CAD build for the part. Positions are in the model's coordinates, mm. Face numbers are marked on the shaded views. A direction names the side the tool comes from. Coordinates: 2 decimals unless noted, no trailing zeros. Loops run counter-clockwise (first coordinate to the right, second up) from the corner with the lowest first, then second, coordinate; pieces in that order, holes last. Notation, with made-up numbers: (-13, -13) - (40, -13) arc R21 ccw to (40, 25) - close; hole circle Ø11 at (-35.75, -5.5). An arc over 180 degrees is marked (long way). Put each result on its own line as item: value.
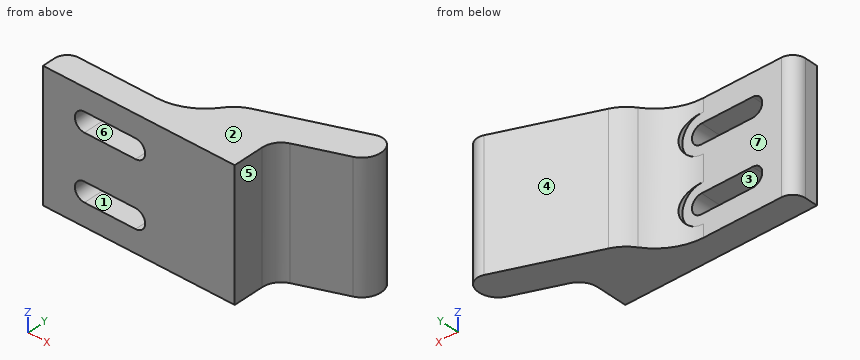
```python
from build123d import *

# Parameters (mm, degrees)
F2_DEPTH = 10
F4_DEPTH = 25
F6_DEPTH = 25


with BuildPart() as f2:
    # F1 (on Top) → F2 (new body, symmetric)
    with BuildSketch(Plane.XY):
        with BuildLine():
            Line((-41.03757, 2), (-41.03757, 0))
            Line((-41.03757, 0), (-11.03757, 0))
            Line((-11.03757, 0), (-11.03757, 4.786366))
            ThreePointArc((-11.03757, 4.786366), (-10.519333, 6.471849), (-9.143667, 7.575012))
            Line((-9.143667, 7.575012), (-1.893904, 10.450577))
            ThreePointArc((-1.893904, 10.450577), (-0.246001, 12.049481), (-0.211353, 14.34532))
            ThreePointArc((-0.211353, 14.34532), (-1.277289, 15.443922), (-2.807848, 15.467021))
            Line((-2.807848, 15.467021), (-17.169758, 9.770475))
            ThreePointArc((-17.169758, 9.770475), (-18.673587, 8.903934), (-19.866468, 7.643207))
            ThreePointArc((-19.866468, 7.643207), (-22.928298, 4.965132), (-26.879931, 4))
            Line((-26.879931, 4), (-39.03757, 4))
            ThreePointArc((-39.03757, 4), (-40.451784, 3.414214), (-41.03757, 2))
        make_face()
    extrude(amount=F2_DEPTH, both=True)

    # F3 (on Front) → F4 (cut)
    with BuildSketch(Plane.XZ):
        with BuildLine():
            ThreePointArc((-34.551002, 6.5), (-36.051002, 5), (-34.551002, 3.5))
            Line((-34.551002, 3.5), (-26.551002, 3.5))
            ThreePointArc((-26.551002, 3.5), (-25.051002, 5), (-26.551002, 6.5))
            Line((-26.551002, 6.5), (-34.551002, 6.5))
        make_face()
        with BuildLine():
            ThreePointArc((-34.551002, -3.5), (-36.051002, -5), (-34.551002, -6.5))
            Line((-34.551002, -6.5), (-26.551002, -6.5))
            ThreePointArc((-26.551002, -6.5), (-25.051002, -5), (-26.551002, -3.5))
            Line((-26.551002, -3.5), (-34.551002, -3.5))
        make_face()
    extrude(amount=-F4_DEPTH, mode=Mode.SUBTRACT)

    # F5 (on face) → F6 (cut)
    with BuildSketch(Plane(origin=(0, 4, 0), x_dir=(-1, 0, 0), z_dir=(0, 1, 0))):
        with BuildLine():
            Line((30.551002, -2), (26.551002, -2))
            ThreePointArc((26.551002, -2), (23.551002, -5), (26.551002, -8))
            Line((26.551002, -8), (30.551002, -8))
            Line((30.551002, -8), (30.551002, -2))
        make_face()
        with BuildLine():
            Line((30.551002, 8), (26.551002, 8))
            ThreePointArc((26.551002, 8), (23.551002, 5), (26.551002, 2))
            Line((26.551002, 2), (30.551002, 2))
            Line((30.551002, 2), (30.551002, 8))
        make_face()
    extrude(amount=F6_DEPTH, mode=Mode.SUBTRACT)


solid = f2.part
```
Q1. Slice it at D-D, the plane y = 3.25. Give the cut face in (x, z), then the cut area to 3 significant figures.
Determined:
outline: (-40.6, -10) - (-11.04, -10) - (-11.04, 10) - (-40.6, 10) - close; hole (-34.55, -6.5) - (-26.55, -6.5) arc R1.5 ccw to (-26.55, -3.5) - (-34.55, -3.5) arc R1.5 ccw to start; hole (-34.55, 3.5) - (-26.55, 3.5) arc R1.5 ccw to (-26.55, 6.5) - (-34.55, 6.5) arc R1.5 ccw to start
area: 529 mm2
Q2. Slice it at B-B, the plane x = -35. Give the cut face in (y, z), then the cut area to 3 significant figures.
Determined:
outline: (0, -10) - (4, -10) - (4, -6.43) - (0, -6.43) - close; (0, -3.57) - (4, -3.57) - (4, 3.57) - (0, 3.57) - close; (0, 6.43) - (4, 6.43) - (4, 10) - (0, 10) - close
area: 57.1 mm2
Q3. Tool access for the marked faces 5, 6 and 7: list every direction of +Z, -Z, +X, -X, +Y, -Y with a clear straight run to the whole face (end or side of a thin tool).
Determined:
face 5: +Z, -Z, +X, -Y
face 6: +Y, -Y
face 7: -X, +Y
Q4. Wall check: L1, parallel to X at y = 1.75, z = 8.5; L2, parallel to Y at x = -30, z = 2; L3, parallel to Y at x = -14.5, z = -2.5. Give the ranges that are in metal, low to high. Write a range as from..to.
Determined:
L1: -41.04..-11.04
L2: 0..4
L3: 0..10.83
Q5. Mould opens along X. For the marked faces 1, 2, 3 and 4 say: +X half, -X half, draft (parallel to the pull), parting line (faces both ways), or undercut.
Determined:
face 1: undercut
face 2: draft
face 3: undercut
face 4: -X half
Q6. Slice it at C-C, the plane z = -0.75. Give the cut face in (x, y), then the cut area to 3 significant figures.
Determined:
outline: (-41.04, 0) - (-11.04, 0) - (-11.04, 4.79) arc R3 cw to (-9.14, 7.58) - (-1.89, 10.45) arc R3 ccw to (-0.21, 14.35) arc R2 ccw to (-2.81, 15.47) - (-17.17, 9.77) arc R6 ccw to (-19.87, 7.64) arc R8.57 cw to (-26.88, 4) - (-39.04, 4) arc R2 ccw to (-41.04, 2) - close
area: 240 mm2
Q7. Slice it at A-A, the plane z = 5. Give the cut face in (x, y).
Determined:
outline: (-41.04, 0) - (-36.05, 0) - (-36.05, 4) - (-39.04, 4) arc R2 ccw to (-41.04, 2) - close; (-25.05, 0) - (-11.04, 0) - (-11.04, 4.79) arc R3 cw to (-9.14, 7.58) - (-1.89, 10.45) arc R3 ccw to (-0.21, 14.35) arc R2 ccw to (-2.81, 15.47) - (-17.17, 9.77) arc R6 ccw to (-19.87, 7.64) arc R8.57 cw to (-23.55, 4.67) - (-23.55, 4) - (-25.05, 4) - close
Q8. Pin check, flat tips, straight feed: pin 1 Ø12 at (x, z) = (-20.5, 2.5) entering from -Y; pin 2 Ø2.5 at (y, z) = (1.5, -2.5) entering from +X; pin 3 Ø8 at (x, z) = (-28, -3) entering from +Y; pin 4 Ø6 at (x, z) = (-13.5, 5.5) entering from +Y. Stop position of each tip, or through.
Determined:
pin 1: y = 0
pin 2: x = -11.04
pin 3: y = 4.5
pin 4: y = 12.42
